from build123d import *

# Parameters (mm, degrees)
SKETCH1_R           = 1.6
BOSS_EXTRUDE1_DEPTH = 9
SKETCH2_R           = 11.1
CUT_EXTRUDE1_DEPTH  = 7
FILLET1_R           = 7
SKETCH3_R           = 6
CUT_EXTRUDE2_DEPTH  = 3


with BuildPart() as part:
    # Sketch1 → Boss-Extrude1 (new body)
    with BuildSketch(Plane(origin=(0, 0, 0), x_dir=(1, 0, 0), z_dir=(0, 1, 0))):
        Polygon((26, 0), (-13, 22.516660498), (-13, -22.516660498), align=None)
        with Locations((-7.5, 12.990381057)):
            Circle(SKETCH1_R, mode=Mode.SUBTRACT)
        with Locations((15, 0)):
            Circle(SKETCH1_R, mode=Mode.SUBTRACT)
        with Locations((-7.5, -12.990381057)):
            Circle(SKETCH1_R, mode=Mode.SUBTRACT)
    extrude(amount=BOSS_EXTRUDE1_DEPTH)

    # Sketch2 → Cut-Extrude1 (cut)
    with BuildSketch(Plane(origin=(0, 9, 0), x_dir=(1, 0, 0), z_dir=(0, 1, 0))):
        Circle(SKETCH2_R)
    extrude(amount=-CUT_EXTRUDE1_DEPTH, mode=Mode.SUBTRACT)

    # Fillet1
    fillet1_edges = [part.edges().sort_by_distance(p)[0] for p in [
        (-13, 4.5, 22.516660498),
        (-13, 4.5, -22.516660498),
        (26, 4.5, 0),
    ]]
    fillet(fillet1_edges, radius=FILLET1_R)

    # Sketch3 → Cut-Extrude2 (cut, through all)
    with BuildSketch(Plane(origin=(0, 2, 0), x_dir=(1, 0, 0), z_dir=(0, 1, 0))):
        Circle(SKETCH3_R)
    extrude(amount=-CUT_EXTRUDE2_DEPTH, mode=Mode.SUBTRACT)


solid = part.part
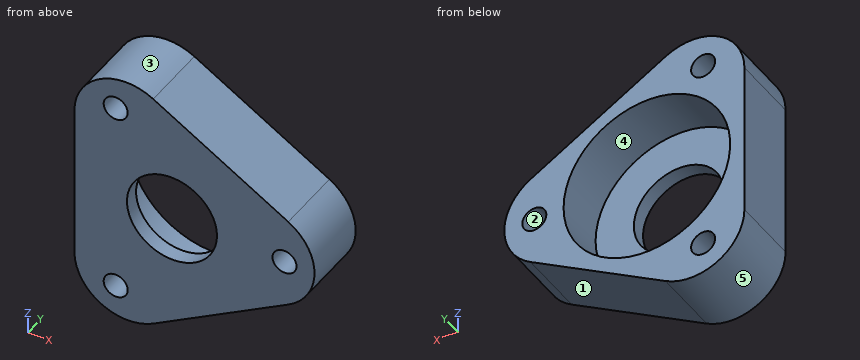
The listing builds one solid part. Answer for the finished solid, in the listing's coordinates (mm). Face numbers are marked on the shaded views. A direction names the side the tool comes from. Round coordinates to 2 decimals unless told otherwise and drop trailing zeros. Order: outer loops, then holes, each group sorted by start corner. A loop starts at its lowest first (then second) coordinate and runs counter-clockwise, first axis right, second up. Notation, with made-up numbers: (64, -21) -> (94, -21) arc R24 ccw to (94, 2) -> close; hole circle Ø9 at (57, 0.25). An arc over 180 degrees is marked (long way). Write each question's results on one line, items separated by ' | '. Start each with the question number.
Q1. The mould has two halves that part along Z. Classify the marked faces 1, 2 and 3: pulls with the +Z half, pulls with the -Z half, needs draft (parallel to the pull), parting line crosses it, or undercut.
Q2. Find section C-C (z = 12.5). Determine the outline of the cut face in (x, y).
Q3. Straight lines are drawn through the part: probe 1 along X at (y, z) = (0.55, 0); probe 2 along X at (y, z) = (4.5, -1); probe 3 along Y at (x, z) = (0, -9.5). For each, find the intervals that lie inside material, in ascending order. Write a range as from..to.
Q4. Which of the six approach directions +Z, -Z, +X, -X, +Y, -Y give full straight-line access (tool end or side, diameter ignored) to the marked faces 4 and 5?
Q5. Find section B-B (x = -7.5). Determine the outline of the cut face in (y, z), then the cut area to 3 significant figures.
Q6. Each of these flat-tipped pins is pushed along its axis until it touches: pin 1 (1.9 mm diameter, centred on x = 15, z = 0, fed in from +Y); pin 2 (1 mm diameter, centred on x = 5, y = 1, fed in from +Z); pin 3 (2 mm diameter, centred on x = 3.5, z = 5, fed in from +Y); pin 4 (4 mm diameter, centred on x = 3.5, y = 5.5, fed in from +Z). Where does it stop, or does it pass through?
Q7. Find section A-A (z = 0). Determine the outline of the cut face in (x, y), then the cut area to 3 significant figures.
Q8. Find section D-D (x = 15). Determine the outline of the cut face in (y, z).
Worked answers:
1) face 1: pulls with the -Z half | face 2: undercut | face 3: pulls with the +Z half
2) outline: (-12.68, 0) -> (-9.02, 0) -> (-9.02, 9) -> (-12.68, 9) -> close; (-5.98, 0) -> (4.35, 0) -> (4.35, 9) -> (-5.98, 9) -> close
3) probe 1: x = -13..-6, 6..13.4, 16.6..19 | probe 2: x = -13..-11.05, 11.05..13.75, 16.25..18.93 | probe 3: y = 0..2
4) face 4: +Y | face 5: -Z, +Y, -Y
5) outline: (0, -17.23) -> (9, -17.23) -> (9, -14.59) -> (0, -14.59) -> close; (0, -11.39) -> (9, -11.39) -> (9, -8.18) -> (2, -8.18) -> (2, 8.18) -> (9, 8.18) -> (9, 11.39) -> (0, 11.39) -> close; (0, 14.59) -> (9, 14.59) -> (9, 17.23) -> (0, 17.23) -> close | area: 138 mm2
6) pin 1: passes through | pin 2: stops at z = 12.41 | pin 3: stops at y = 2 | pin 4: stops at z = 14.15
7) outline: (-13, 0) -> (-6, 0) -> (-6, 2) -> (-11.1, 2) -> (-11.1, 9) -> (-13, 9) -> close; (6, 0) -> (13.4, 0) -> (13.4, 9) -> (11.1, 9) -> (11.1, 2) -> (6, 2) -> close; (16.6, 0) -> (19, 0) -> (19, 9) -> (16.6, 9) -> close | area: 79.8 mm2
8) outline: (0, -6.35) -> (9, -6.35) -> (9, -1.6) -> (0, -1.6) -> close; (0, 1.6) -> (9, 1.6) -> (9, 6.35) -> (0, 6.35) -> close
